Part print with two shaded views. Sizes in mm from the minimum x, y, z corner. A direction names the side the tool comes from. Coordinates: 2 decimals unless noted, no trailing zeros. Order: outer loops, then holes, each group sorted by start corner. A loop starts at its lowest first (then second) coordinate and runs counter-clockwise, first axis right, second up. Notation, with made-up numbers: M 38.5,33.5 L 57.5,33.5 A34 cw 57.5,72.5 Z; hole C 21.5,-32 d2. An arc over 180 degrees is marked long. Answer in a Markdown table with one row per item. Add a question column.
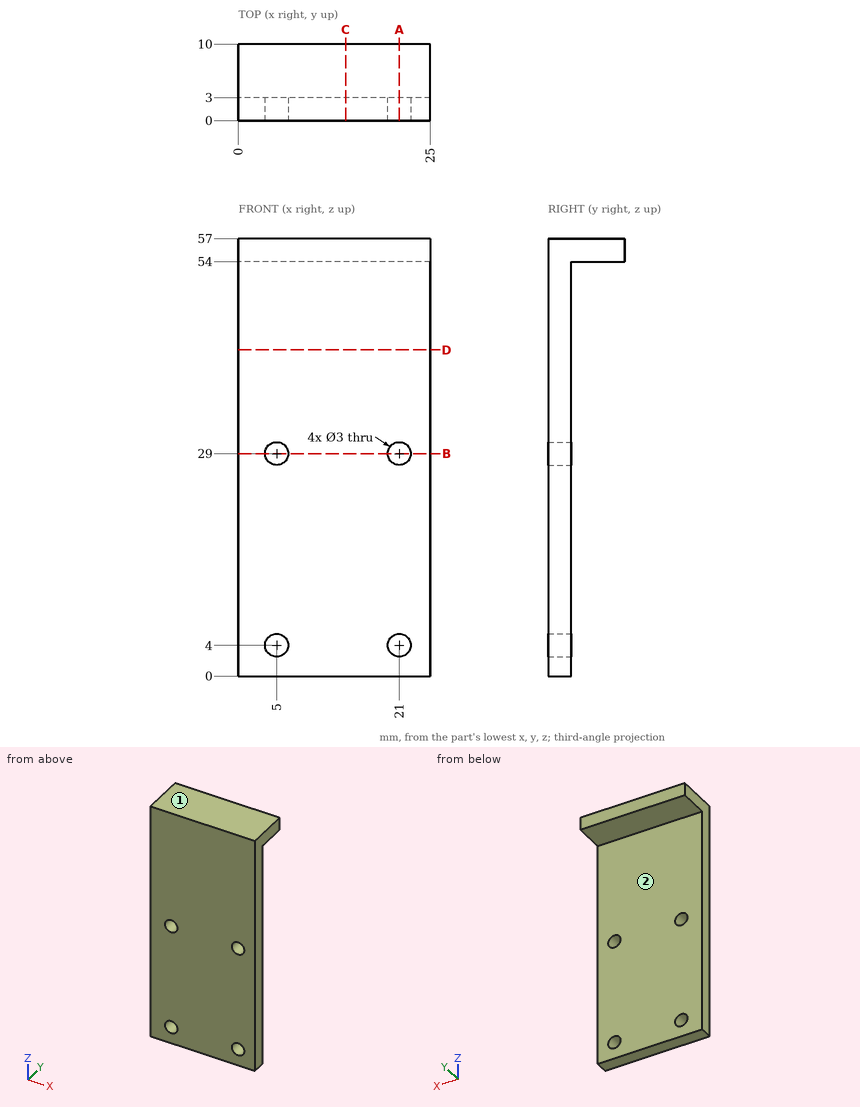
(1) Slice it at B-B (z = 29). List the corners of the cut face in (x, y).
(2) Drop flat-ended pins along their axis: P1, Ø4, axis at x = 10.5, y = 6, coming from the -Z side; P2, Ø8, axis at x = 8, z = 7, coming from the -Y side; P3, Ø10, axis at x = 18.5, z = 20.5, coming from the +Y side. Give the stop position or say it passes through.
(3) Wall check: line 1 (X direction, y = 2.3, z = 4); line 2 (Z direction, x = 21, y = 1.45); line 3 (Y direction, x = 15, z = 52.5). Give the ranges that are in metal, low to high.
(4) Slice it at D-D (z = 42.5). List the corners of the cut face in (x, y), and give its area (3 significant figures).
(5) 3-axis set-ups, long thin cutter, end or side, ignore diameter. For the marked faces 1 and 2: which of +Z, -Z, +X, -X, +Y, -Y reach the whole face in a straight line?
(6) Slice it at C-C (x = 14). List the corners of the cut face in (y, z), and give its area (3 significant figures).
(7) Slice it at A-A (x = 21). List the corners of the cut face in (y, z).
Computed:
| question | item | result |
|---|---|---|
| 1 | outline | M 0,0 L 3.5,0 L 3.5,3 L 0,3 Z; M 6.5,0 L 19.5,0 L 19.5,3 L 6.5,3 Z; M 22.5,0 L 25,0 L 25,3 L 22.5,3 Z |
| 2 | P1 | stops at z = 54 |
| 2 | P2 | stops at y = 0 |
| 2 | P3 | stops at y = 3 |
| 3 | line 1 | x = 0 to 3.5, 6.5 to 19.5, 22.5 to 25 |
| 3 | line 2 | z = 0 to 2.5, 5.5 to 27.5, 30.5 to 57 |
| 3 | line 3 | y = 0 to 3 |
| 4 | outline | M 0,0 L 25,0 L 25,3 L 0,3 Z |
| 4 | area | 75.0 mm^2 |
| 5 | face 1 | +Z, +X, -X, +Y, -Y |
| 5 | face 2 | -Z, +X, -X, +Y |
| 6 | outline | M 0,0 L 3,0 L 3,54 L 10,54 L 10,57 L 0,57 Z |
| 6 | area | 192 mm^2 |
| 7 | outline | M 0,0 L 3,0 L 3,2.5 L 0,2.5 Z; M 0,5.5 L 3,5.5 L 3,27.5 L 0,27.5 Z; M 0,30.5 L 3,30.5 L 3,54 L 10,54 L 10,57 L 0,57 Z |
